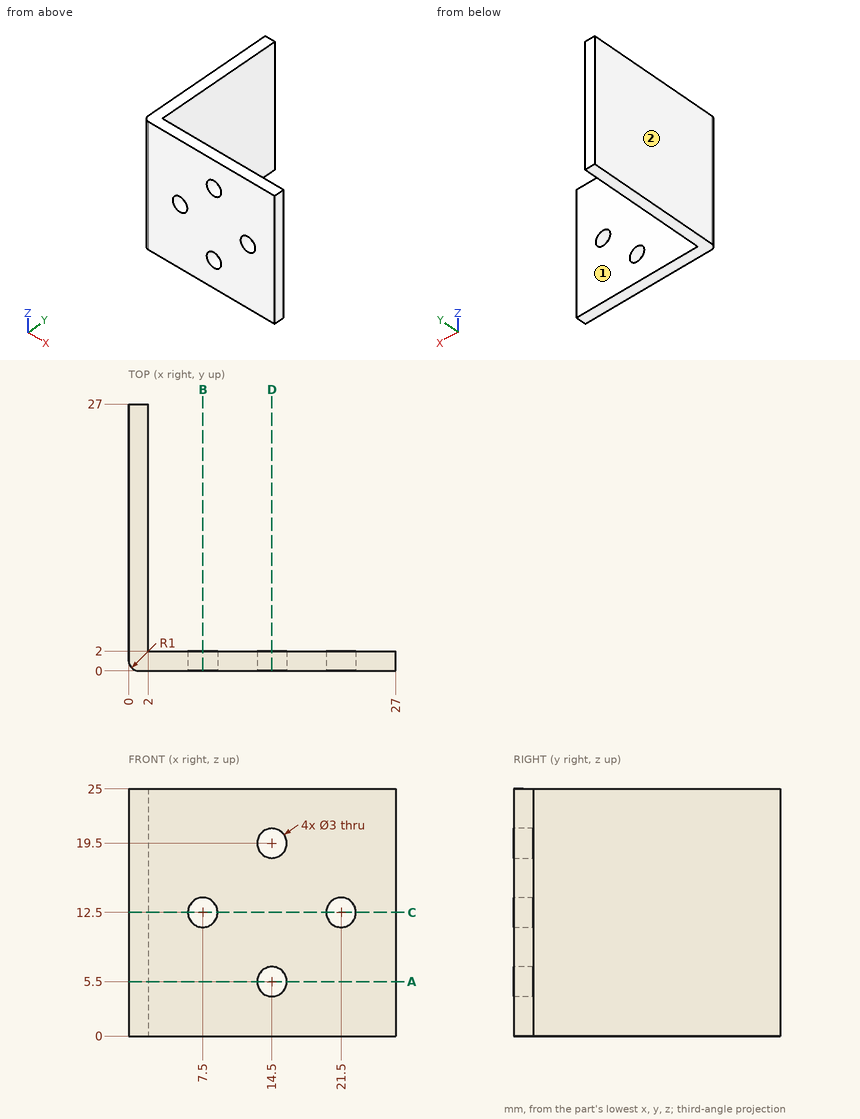
Geometry check sheet. Reference: drawing and pictorial views, mm from the part's lowest x, y, z. A direction names the side the tool comes from. Coordinates: 2 decimals unless noted, no trailing zeros. Order: outer loops, then holes, each group sorted by start corner. A loop starts at its lowest first (then second) coordinate and runs counter-clockwise, first axis right, second up. Notation, with made-up numbers: (43, 47.25) -> (53, 47.25) arc R24 ccw to (53, 73.25) -> close; hole circle Ø8 at (67.5, 77). An arc over 180 degrees is marked (long way). Put each result on its own line as item: value. Start each with the question number.
1) Cross-section at A-A (z = 5.5). Enter the section's corners in (x, y).
2) Cross-section at B-B (x = 7.5). Enter the section's corners in (y, z), plus the area to 3 significant figures.
3) Cross-section at C-C (z = 12.5). Enter the section's corners in (x, y).
4) Cross-section at D-D (x = 14.5). Enter the section's corners in (y, z).
5) Material ranges on L1, parallel to X at y = 1.15, z = 12.5; L2, parallel to X at y = 1.3, z = 5.5; L3, parallel to Y at x = 15, z = 14.25, recorded low to high.
6) Go/stop test with flat-tipped pins: pin 1 (8 mm diameter, centred on x = 14, y = 8.5, fed in from -Z); pin 2 (3.5 mm diameter, centred on x = 7.5, z = 12.5, fed in from +Y); pin 3 (1.5 mm diameter, centred on y = 23, z = 13.5, fed in from +X). Record where each tip stops, or that it passes through.
7) Tool access check on the marked faces 1 and 2. Record the directions out of +Z, -Z, +X, -X, +Y, -Y that give a thin tool (end or side, any length) a straight path to the whole face; none if there is none.
Geometry check:
1. outline: (0, 1) arc R1 ccw to (1, 0) -> (13, 0) -> (13, 2) -> (2, 2) -> (2, 27) -> (0, 27) -> close; (16, 0) -> (27, 0) -> (27, 2) -> (16, 2) -> close
2. outline: (0, 0) -> (2, 0) -> (2, 11) -> (0, 11) -> close; (0, 14) -> (2, 14) -> (2, 25) -> (0, 25) -> close
2. area: 44.0 mm^2
3. outline: (0, 1) arc R1 ccw to (1, 0) -> (6, 0) -> (6, 2) -> (2, 2) -> (2, 27) -> (0, 27) -> close; (9, 0) -> (20, 0) -> (20, 2) -> (9, 2) -> close; (23, 0) -> (27, 0) -> (27, 2) -> (23, 2) -> close
4. outline: (0, 0) -> (2, 0) -> (2, 4) -> (0, 4) -> close; (0, 7) -> (2, 7) -> (2, 18) -> (0, 18) -> close; (0, 21) -> (2, 21) -> (2, 25) -> (0, 25) -> close
5. L1: x = 0 to 6, 9 to 20, 23 to 27
5. L2: x = 0 to 13, 16 to 27
5. L3: y = 0 to 2
6. pin 1: passes through
6. pin 2: stops at y = 2
6. pin 3: stops at x = 2
7. face 1: +Z, -Z, +X, +Y
7. face 2: +Z, -Z, -X, +Y, -Y
